Work out the finished part from the listing and answer in its coordinate system (mm). Round coordinates to 2 decimals unless told otherwise and drop trailing zeros. Order: outer loops, then holes, each group sorted by start corner. A loop starts at its lowest first (then second) coordinate and runs counter-clockwise, first axis right, second up. Notation, with made-up numbers: (89, 59) - (115, 59) arc R14 ccw to (115, 82) - close; hole circle Ø1 at (8, -3.5). An arc over 180 degrees is marked (long way). Use CSV: the item, a comma, the result in double quotes.
from build123d import *

# Parameters (mm, degrees)
BOSS_EXTRU_1_DEPTH      = 2.5
ESQUISSE21_W            = 15
ESQUISSE21_H            = 15
ENL_V_MAT_EXTRU_1_DEPTH = 10


with BuildPart() as part:
    # Esquisse20 → Boss.-Extru.1 (new body)
    with BuildSketch(Plane.XY):
        with BuildLine():
            Line((14.8, -2), (164.37, -2))
            ThreePointArc((164.37, -2), (174.835180362, 2.334819638), (179.17, 12.8))
            Line((179.17, 12.8), (179.17, 57.73))
            ThreePointArc((179.17, 57.73), (177.851980515, 60.911980515), (174.67, 62.23))
            Line((174.67, 62.23), (4.5, 62.23))
            ThreePointArc((4.5, 62.23), (1.318019485, 60.911980515), (0, 57.73))
            Line((0, 57.73), (0, 12.8))
            ThreePointArc((0, 12.8), (4.334819638, 2.334819638), (14.8, -2))
        make_face()
    extrude(amount=BOSS_EXTRU_1_DEPTH)

    # Esquisse21 → Enlèv. mat.-Extru.1 (cut)
    with BuildSketch(Plane(origin=(0, 0, 0), x_dir=(-1, 0, 0), z_dir=(0, 0, -1))):
        with Locations((-130.294905016, 13.280151044)):
            Rectangle(ESQUISSE21_W, ESQUISSE21_H)
    extrude(amount=-ENL_V_MAT_EXTRU_1_DEPTH, mode=Mode.SUBTRACT)


solid = part.part
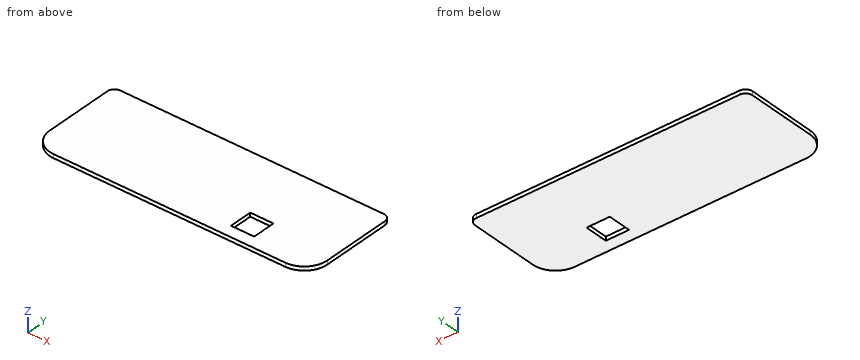
(1) Find section B-B (x = 130). Determine the outline of the cut face in (y, z), and give its area (3 significant figures).
Findings below:
outline,"(-2, 0) - (5.78, 0) - (5.78, 2.5) - (-2, 2.5) - close; (20.78, 0) - (62.23, 0) - (62.23, 2.5) - (20.78, 2.5) - close"
area,"123 mm²"
(2) Find section C-C (z = 1.7). Determine the outline of the cut face in (x, y).
Findings below:
outline,"(0, 12.8) arc R14.8 ccw to (14.8, -2) - (164.37, -2) arc R14.8 ccw to (179.17, 12.8) - (179.17, 57.73) arc R4.5 ccw to (174.67, 62.23) - (4.5, 62.23) arc R4.5 ccw to (0, 57.73) - close; hole (122.79, 5.78) - (137.79, 5.78) - (137.79, 20.78) - (122.79, 20.78) - close"
(3) Find section A-A (y = 17). Determine the outline of the cut face in (x, z), and give its area (3 significant figures).
Findings below:
outline,"(0, 0) - (122.79, 0) - (122.79, 2.5) - (0, 2.5) - close; (137.79, 0) - (179.17, 0) - (179.17, 2.5) - (137.79, 2.5) - close"
area,"410 mm²"
(4) Find the intervals of material crossed by L1, parallel to X at y = 19.5, z = 0.7; L2, parallel to Y at x = 135, z = 1.4; L3, parallel to X at y = 6.5, z = 1.3, in increasing order. Write a range as from..to.
Findings below:
L1,"x = 0..122.79, 137.79..179.17"
L2,"y = -2..5.78, 20.78..62.23"
L3,"x = 1.41..122.79, 137.79..177.76"
